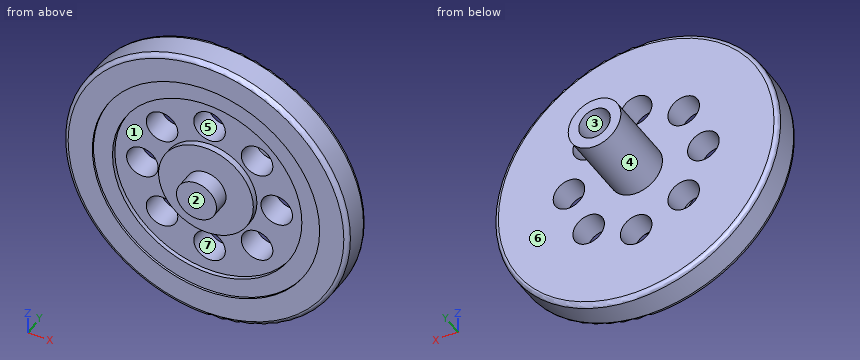
```python
from build123d import *

# Parameters (mm, degrees)
F0_R      = 17.145
F1_DEPTH  = 3.81
F2_R      = 13.716
F2_R_2    = 11.43
F3_DEPTH  = 0.254
F4_DEPTH  = 0.762
F5_R      = 5.715
F6_DEPTH  = 0.762
F8_R      = 1.905
F9_DEPTH  = 25.4
F10_R     = 2.413
F11_DEPTH = 2.032
F14_R     = 3.175
F15_DEPTH = 8.89
F16_R     = 1.905
F17_DEPTH = 8.89
F18_R     = 0.508
F19_R     = 0.508


# Not quite as in the source:
# - the program builds the solid bodies; features that only make, move or delete a surface that nothing else refers to are left out


with BuildPart() as f1:
    # F0 (on Front) → F1 (new body)
    with BuildSketch(Plane.XZ):
        Circle(F0_R)
    extrude(amount=F1_DEPTH)

    # F2 (on face) → F3 (cut)
    with BuildSketch(Plane.XZ.offset(3.81)):
        Circle(F2_R)
        Circle(F2_R_2, mode=Mode.SUBTRACT)
    extrude(amount=-F3_DEPTH, mode=Mode.SUBTRACT)

    # F4 (cut): a face of the model
    f4_faces = [f1.faces().sort_by_distance(p)[0] for p in [
        (0, -3.81, 0),
    ]]
    extrude(f4_faces, amount=-F4_DEPTH, mode=Mode.SUBTRACT)

    # F5 (on face) → F6 (join)
    with BuildSketch(Plane.XZ.offset(3.048)):
        Circle(F5_R)
    extrude(amount=F6_DEPTH)

    # F8 (on face) → F9 (cut)
    with BuildSketch(Plane.XZ.offset(3.048)):
        with Locations((0, 8.1100180022)):
            Circle(F8_R)
        with Locations((-5.7346487249, 5.7346487249)):
            Circle(F8_R)
        with Locations((-5.7346487249, -5.7346487249)):
            Circle(F8_R)
        with Locations((0, -8.1100180022)):
            Circle(F8_R)
        with Locations((5.7346487249, -5.7346487249)):
            Circle(F8_R)
        with Locations((8.1100180022, 0)):
            Circle(F8_R)
        with Locations((5.7346487249, 5.7346487249)):
            Circle(F8_R)
        with Locations((-8.1100180022, 0)):
            Circle(F8_R)
    extrude(amount=-F9_DEPTH, mode=Mode.SUBTRACT)

    # F10 (on face) → F11 (join)
    with BuildSketch(Plane.XZ.offset(3.81)):
        Circle(F10_R)
    extrude(amount=F11_DEPTH)

    # F14 (on Front) → F15 (join)
    with BuildSketch(Plane.XZ):
        Circle(F14_R)
    extrude(amount=-F15_DEPTH)

    # F16 (on face) → F17 (cut)
    with BuildSketch(Plane(origin=(0, 8.89, 0), x_dir=(-1, 0, 0), z_dir=(0, 1, 0))):
        Circle(F16_R)
    extrude(amount=-F17_DEPTH, mode=Mode.SUBTRACT)

    # F18
    f18_edges = [f1.edges().sort_by_distance(p)[0] for p in [
        (-17.145, -3.81, 0),
    ]]
    fillet(f18_edges, radius=F18_R)

    # F19
    f19_edges = [f1.edges().sort_by_distance(p)[0] for p in [
        (-17.145, 0, 0),
    ]]
    fillet(f19_edges, radius=F19_R)


solid = f1.part
```
Geometry: final body of the model. Coordinates: model frame, mm. Face numbers are marked on the shaded views. A direction names the side the tool comes from. Give positions to 0.01 mm unless a question says otherwise; leave off trailing zeros. Order: outer loops, then holes, each group sorted by start corner. A loop starts at its lowest first (then second) coordinate and runs counter-clockwise, first axis right, second up. Notation, with made-up numbers: (81, 36.5) -> (88, 36.5) arc R16 cw to (88, 67.5) -> close; hole circle Ø5 at (14, 47.5). An arc over 180 degrees is marked (long way). Write each question's results on one line, items separated by ' | '. Start each with the question number.
1) Draft query along X for the marked faces 4, 5, 6 and 7. Return one class per face: pulls with the +X half, pulls with the -X half, needs draft (parallel to the pull), parting line crosses it, or undercut.
2) Section A-A (x = 0). Count the separate pieces of the cut face and the enclosed holes in it, then the cut area to 3 significant figures.
3) Line query: line 1 (Z direction, x = 0, y = -2.1) (3 decimals); line 2 (Z direction, x = 0, y = -3.25) (3 decimals); line 3 (X direction, y = -1, z = -6.5). Output: solid intervals per line, ascending. Write a range as from..to.
4) Set-up query: the marked faces 1, 2 and 3. Return all of +Z, -Z, +X, -X, +Y, -Y with unobstructed straight access to the full face (end or side cutting, diameter ignored); none if empty.
5) Section B-B (y = 6.25). Return loops of the section in (x, z) (3 decimals), then the cut area to 3 significant figures.
6) First-contact query: pin 1 (4.5 mm diameter, centred on x = -5.73, z = 5.73, fed in from +Y); pin 2 (6 mm diameter, centred on x = 5.73, z = -5.73, fed in from -Y); pin 3 (6 mm diameter, centred on y = -3.5, z = -10.5, fed in from +X); pin 4 (1.5 mm diameter, centred on x = -6, y = 1.5, fed in from -Z). Flat tips, straight axial feed; report the tip coordinate or a pass-through.
Calculated:
1) face 4: parting line crosses it | face 5: undercut | face 6: needs draft | face 7: undercut
2) separate pieces: 3 | enclosed holes: 0 | area: 130 mm2
3) line 1: -17.145..-10.015, -6.205..6.205, 10.015..17.145 | line 2: -17.145..-11.43, -5.715..5.715, 11.43..17.145 | line 3: -15.87..-7.48, -3.99..-1.02, 1.02..3.99, 7.48..15.87
4) face 1: -Y | face 2: +Z, -Z, +X, -X, -Y | face 3: +Y
5) outline: circle Ø6.35 at (0, 0); hole circle Ø3.81 at (0, 0) | area: 20.3 mm2
6) pin 1: y = 0 | pin 2: y = -3.81 | pin 3: x = 15.41 | pin 4: through
